Check sheet for the modelled part. Datum: model origin and axes. Units: mm. Face numbers are marked on the shaded views. A direction names the side the tool comes from. Round coordinates to 2 decimals unless told otherwise and drop trailing zeros. Write each loop counter-clockwise with the first axis right and the second up, starting at its lowest first coordinate (ties: lowest second). Pieces come first, ordered by that corner, then holes. Notation, with made-up numbers: (39, 17) - (82, 17) arc R26 cw to (82, 49) - close; hole circle Ø6 at (40, -20.75). An arc over 180 degrees is marked (long way). Answer as a JSON object with one key per item and string values. Group by question number.
Item 1: Release check for a two-part mould opening along X. For the marked faces 4, 5, 6 and 7 record: pulls with the +X half, pulls with the -X half, needs draft (parallel to the pull), parting line crosses it, or undercut.
Item 2: Set-up check for the marked faces 1, 2 and 3: record each of +Z, -Z, +X, -X, +Y, -Y from which the full face is reachable in a straight line by a thin tool's end or side.
Item 3: Gauge pin test, flat ends, axial feed: P1, Ø1, axis at y = -464, z = -316, coming from the +X side; P2, Ø8, axis at y = -104.5, z = -256, coming from the -X side; P3, Ø1.5, axis at x = -799, y = -194.5, coming from the +Z side. Record the tip position at first contact, or that the pin passes through.
Item 4: Sectioned sample at A-A on y = -434.5. Record the boundary of the cut face in (x, z), plus the area to 3 significant figures.
Item 5: Thickness scan on line 1 (Z direction, x = -1220.5, y = -165); line 2 (X direction, y = -584, z = 65.5); line 3 (X direction, y = -61.5, z = -76.5). Record the ranges inside material, lowest first.
Item 6: Sectioned sample at B-B on x = 130. Record the boundary of the cut face in (y, z), plus the area to 4 significant figures.
Item 7: Sectioned sample at C-C on x = -400. Record the boundary of the cut face in (y, z), plus the area to 3 significant figures.
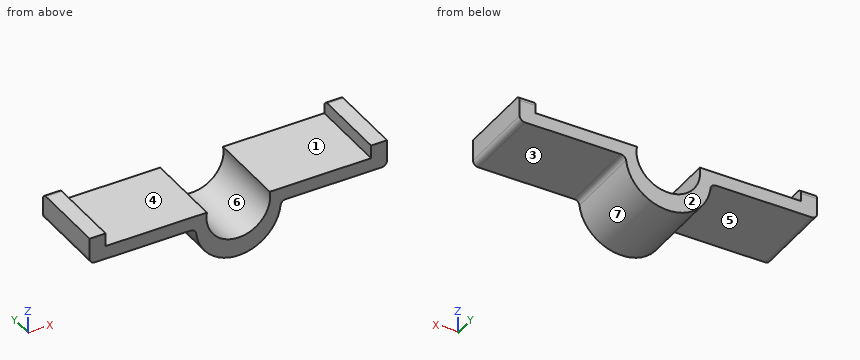
```python
from build123d import *

# Parameters (mm, degrees)
F1_DEPTH = 750
F2_R     = 50
F3_R     = 50
F4_R     = 50
F5_R     = 50
F6_R     = 50


with BuildPart() as f1:
    # F0 (on Front) → F1 (new body)
    with BuildSketch(Plane.XZ):
        with BuildLine():
            ThreePointArc((-800, 0), (-400, -400), (0, 0))
            Line((0, 0), (1000, 0))
            Line((1000, 0), (1000, 250))
            Line((1000, 250), (850, 250))
            Line((850, 250), (850, 125))
            Line((850, 125), (-104.070191, 125))
            ThreePointArc((-104.070191, 125), (-400, -224.249854), (-695.929809, 125))
            Line((-695.929809, 125), (-1650, 125))
            Line((-1650, 125), (-1650, 250))
            Line((-1650, 250), (-1800, 250))
            Line((-1800, 250), (-1800, 0))
            Line((-1800, 0), (-800, 0))
        make_face()
    extrude(amount=F1_DEPTH)

    # F2
    f2_edges = [f1.edges().sort_by_distance(p)[0] for p in [
        (1000, -375, 0),
    ]]
    fillet(f2_edges, radius=F2_R)

    # F3
    f3_edges = [f1.edges().sort_by_distance(p)[0] for p in [
        (925, 0, 250),
    ]]
    fillet(f3_edges, radius=F3_R)

    # F4
    f4_edges = [f1.edges().sort_by_distance(p)[0] for p in [
        (0, -375, 0),
    ]]
    fillet(f4_edges, radius=F4_R)

    # F5
    f5_edges = [f1.edges().sort_by_distance(p)[0] for p in [
        (-800, -375, 0),
    ]]
    fillet(f5_edges, radius=F5_R)

    # F6
    f6_edges = [f1.edges().sort_by_distance(p)[0] for p in [
        (-1800, -375, 0),
        (-1725, 0, 250),
    ]]
    fillet(f6_edges, radius=F6_R)


solid = f1.part
```
Completed:
{
 "1": {"face 4": "undercut", "face 5": "needs draft", "face 6": "undercut", "face 7": "parting line crosses it"},
 "2": {"face 1": "+Z, +Y, -Y", "face 2": "+Z, -Z, +X, -X, +Y", "face 3": "-Z, +X, +Y, -Y"},
 "3": {"P1": "x = -154.11", "P2": "x = -710.64", "P3": "z = 125"},
 "4": {"outline": "(-1800, 50) arc R50 ccw to (-1750, 0) - (-847.21, 0) arc R50 cw to (-797.52, -44.44) arc R400 ccw to (-2.48, -44.44) arc R50 cw to (47.21, 0) - (950, 0) arc R50 ccw to (1000, 50) - (1000, 250) - (850, 250) - (850, 125) - (-104.07, 125) arc R300 cw (long way) to (-695.93, 125) - (-1650, 125) - (-1650, 250) - (-1800, 250) - close", "area": "468,000 mm²"},
 "5": {"line 1": "0 to 125", "line 2": "-1800 to -699.82, -100.18 to 1000", "line 3": "-792.62 to -658.5, -141.5 to -7.38"},
 "6": {"outline": "(-750, 0) - (0, 0) - (0, 125) - (-750, 125) - close", "area": "93,750 mm²"},
 "7": {"outline": "(-750, -400) - (0, -400) - (0, -224.25) - (-750, -224.25) - close", "area": "132,000 mm²"}
}
